Here's how the part is built. I have some questions about the finished solid (model axes, mm). A direction names the side the tool comes from. Coordinates: 2 decimals unless noted, no trailing zeros. Write each loop counter-clockwise with the first axis right and the second up, starting at its lowest first coordinate (ties: lowest second). Pieces come first, ordered by that corner, then holes. Notation, with made-up numbers: (55.25, -14) - (90.25, -14) arc R27 ccw to (90.25, 4) - close; hole circle Ø6 at (70.5, 5.5). An arc over 180 degrees is marked (long way). Answer in a Markdown table with one row per item. Add a question column.
Item 1: Imagine slicing it at B-B (z = 34). Please give me the cut outline in (x, y).
Item 2: Imagine slicing it at A-A (y = 0). Please give me the cut outline in (x, z), plus the area to 3 significant figures.
Item 3: We'd pull the mould along X, two halves only. Please class faces 1 (the face through (0, -7.5, 19)), 2 (the face through (-0.867, -3.905, 18.734)), 3 (the face through (15, 0, 19)): +X half, -X half, draft (parallel to the pull), parting line (faces both ways), or undercut.
Item 4: Imagine slicing it at D-D (y = 3.5). State how many separate pieces and enclosed holes the cut face has, plus the area to 3 significant figures.
Item 5: I'm going to push a flat-ended pin straight in: pin 1 (2.5 mm diameter, centred on x = 9, z = 11, fed in from +Y). Where does the tip first touch, or does it pass through?
Item 6: Which directions (+Z, -Z, +X, -X, +Y, -Y) give clear straight access to the entire face, cutting with the end or side of a thin tool? Please do faces 4 (the face through (-15, 0, 19)), 5 (the face through (10, 1.5, 34)).
Item 7: Imagine slicing it at C-C (x = -10). Please give me the cut outline in (y, z), plus the area to 3 significant figures.
Item 8: If I drill on probe 1 along X at (y, z) = (5.3, 19); probe 2 along X at (y, z) = (4.05, 11.5); probe 3 along X at (y, z) = (-0.25, 36.5), over which ranges is the centre line in solid material (lowest first)? Write a range as from..to.
from build123d import *

# Parameters (mm, degrees)
SKETCH_1_W          = 30
SKETCH_1_H          = 15
SKETCH_1_R          = 4
EXTRUDE_1_DEPTH     = 38
SKETCH_2_R          = 2
SKETCH_2_R_2        = 2.5
CUT_EXTRUDE_1_DEPTH = 6


with BuildPart() as part:
    # 草图1 → 凸台-拉伸1 (new body)
    with BuildSketch(Plane.XY):
        Rectangle(SKETCH_1_W, SKETCH_1_H)
        Circle(SKETCH_1_R, mode=Mode.SUBTRACT)
    extrude(amount=EXTRUDE_1_DEPTH)

    # 草图2 → 切除-拉伸1 (cut)
    with BuildSketch(Plane(origin=(0, 7.5, 0), x_dir=(1, 0, 0), z_dir=(0, 1, 0))):
        with Locations(Location((10, -19, 0), (0, 0, 270))):
            Circle(SKETCH_2_R)
        with Locations(Location((-10, -19, 0), (0, 0, 270))):
            Circle(SKETCH_2_R)
        with Locations(Location((10, -26.5, 0), (0, 0, 270))):
            Circle(SKETCH_2_R_2)
        with Locations(Location((-10, -26.5, 0), (0, 0, 270))):
            Circle(SKETCH_2_R_2)
        with Locations(Location((-10, -34, 0), (0, 0, 270))):
            Circle(SKETCH_2_R)
        with Locations(Location((10, -34, 0), (0, 0, 270))):
            Circle(SKETCH_2_R)
        with Locations(Location((10, -11.5, 0), (0, 0, 270))):
            Circle(SKETCH_2_R_2)
        with Locations(Location((-10, -11.5, 0), (0, 0, 270))):
            Circle(SKETCH_2_R_2)
    extrude(amount=-CUT_EXTRUDE_1_DEPTH, mode=Mode.SUBTRACT)


solid = part.part
Here are the results:
| question | item | result |
|---|---|---|
| 1 | outline | (-15, -7.5) - (15, -7.5) - (15, 7.5) - (12, 7.5) - (12, 1.5) - (8, 1.5) - (8, 7.5) - (-8, 7.5) - (-8, 1.5) - (-12, 1.5) - (-12, 7.5) - (-15, 7.5) - close; hole circle Ø8 at (0, 0) |
| 2 | outline | (-15, 0) - (-4, 0) - (-4, 38) - (-15, 38) - close; (4, 0) - (15, 0) - (15, 38) - (4, 38) - close |
| 2 | area | 836 mm2 |
| 3 | face 1 | draft |
| 3 | face 2 | undercut |
| 3 | face 3 | +X half |
| 4 | separate pieces | 2 |
| 4 | enclosed holes | 8 |
| 4 | area | 864 mm2 |
| 5 | pin 1 | stops at y = 1.5 |
| 6 | face 4 | +Z, -Z, -X, +Y, -Y |
| 6 | face 5 | +Y |
| 7 | outline | (-7.5, 0) - (7.5, 0) - (7.5, 9) - (1.5, 9) - (1.5, 14) - (7.5, 14) - (7.5, 17) - (1.5, 17) - (1.5, 21) - (7.5, 21) - (7.5, 24) - (1.5, 24) - (1.5, 29) - (7.5, 29) - (7.5, 32) - (1.5, 32) - (1.5, 36) - (7.5, 36) - (7.5, 38) - (-7.5, 38) - close |
| 7 | area | 462 mm2 |
| 8 | probe 1 | x = -15..-12, -8..8, 12..15 |
| 8 | probe 2 | x = -15..-12.5, -7.5..7.5, 12.5..15 |
| 8 | probe 3 | x = -15..-3.99, 3.99..15 |
